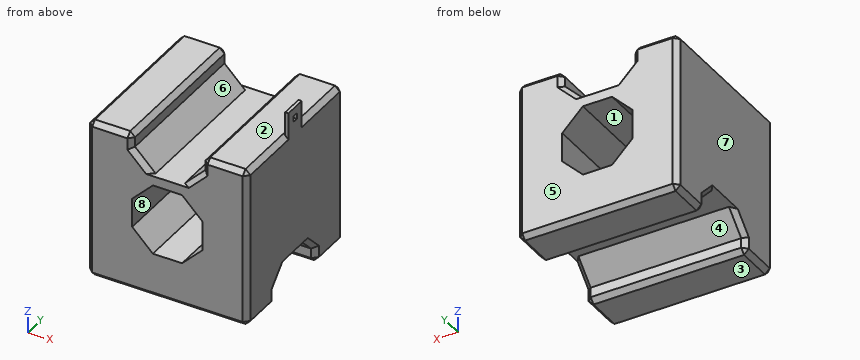
```python
from build123d import *

# Parameters (mm, degrees)
SKETCH1_W                = 50
SKETCH1_H                = 50
BOSS_EXTRUDE1_DEPTH      = 50
CUT_EXTRUDE2_DEPTH       = 87.602540378
CUT_EXTRUDE3_DEPTH       = 87.602540378
CHAMFER1_SIZE            = 1.5
BOSS_EXTRUDE2_DEPTH      = 7
BOSS_EXTRUDE2_DEPTH_BACK = 10
SKETCH5_W                = 1
SKETCH5_H                = 7
SKETCH6_W                = 1.8
SKETCH6_H                = 1.8
CUT_EXTRUDE4_DEPTH       = 7


with BuildPart() as part:
    # Sketch1 → Boss-Extrude1 (new body)
    with BuildSketch(Plane.XY):
        with Locations((25, 25)):
            Rectangle(SKETCH1_W, SKETCH1_H)
    extrude(amount=BOSS_EXTRUDE1_DEPTH)

    # Sketch3 → Cut-Extrude2 (cut, through all)
    with BuildSketch(Plane.XZ):
        Polygon((29.556349186, 36), (20.443650814, 36), (14, 29.556349186), (14, 20.443650814), (20.443650814, 14), (29.556349186, 14), (36, 20.443650814), (36, 29.556349186), align=None)
        Polygon((29.556349186, 39), (36, 45.443650814), (36, 54.556349186), (29.556349186, 61), (20.443650814, 61), (14, 54.556349186), (14, 45.443650814), (20.443650814, 39), align=None)
    extrude(amount=-CUT_EXTRUDE2_DEPTH, mode=Mode.SUBTRACT)

    # Sketch4 → Cut-Extrude3 (cut, through all)
    with BuildSketch(Plane.ZY):
        Polygon((4.556349186, 14), (11, 20.443650814), (11, 29.556349186), (4.556349186, 36), (-4.556349186, 36), (-11, 29.556349186), (-11, 20.443650814), (-4.556349186, 14), align=None)
    extrude(amount=-CUT_EXTRUDE3_DEPTH, mode=Mode.SUBTRACT)

    # Chamfer1
    chamfer1_edges = [part.edges().sort_by_distance(p)[0] for p in [
        (50, 25, 50),
        (43, 50, 50),
        (43, 0, 50),
        (7, 50, 50),
        (36, 25, 50),
        (14, 25, 50),
        (0, 25, 50),
        (14, 50, 47.721825407),
        (36, 50, 47.721825407),
        (25, 50, 0),
        (36, 0, 47.721825407),
        (14, 0, 47.721825407),
        (17.221825407, 0, 42.221825407),
        (32.778174593, 0, 42.221825407),
        (17.221825407, 50, 42.221825407),
        (50, 7, 0),
        (32.778174593, 50, 42.221825407),
        (25, 0, 0),
        (0, 43, 0),
        (7, 0, 50),
        (0, 50, 25),
        (50, 50, 25),
        (50, 0, 25),
        (0, 0, 25),
        (0, 7, 0),
        (50, 43, 0),
        (25, 36, 0),
        (25, 14, 0),
        (50, 14, 2.278174593),
        (50, 36, 2.278174593),
        (50, 32.778174593, 7.778174593),
        (50, 17.221825407, 7.778174593),
        (0, 14, 2.278174593),
        (0, 17.221825407, 7.778174593),
        (0, 32.778174593, 7.778174593),
        (0, 36, 2.278174593),
    ]]
    chamfer(chamfer1_edges, length=CHAMFER1_SIZE)

    # Sketch5 → Boss-Extrude2 (add, two sides: drawn at the far end of the back side and taken through both)
    with BuildSketch(Plane.XY.offset(50).offset(-BOSS_EXTRUDE2_DEPTH_BACK)):
        with Locations((49.5, 25)):
            Rectangle(SKETCH5_W, SKETCH5_H)
    extrude(amount=BOSS_EXTRUDE2_DEPTH + BOSS_EXTRUDE2_DEPTH_BACK)

    # Sketch6 → Cut-Extrude4 (cut)
    with BuildSketch(Plane(origin=(50, 0, 0), x_dir=(0, 0, -1), z_dir=(1, 0, 0))):
        with Locations((-53.6, 25)):
            Rectangle(SKETCH6_W, SKETCH6_H)
    extrude(amount=-CUT_EXTRUDE4_DEPTH, mode=Mode.SUBTRACT)


solid = part.part
```
Work out the finished part from the listing and answer in its coordinate system (mm). Face numbers are marked on the shaded views. A direction names the side the tool comes from. Give positions to 0.01 mm unless a question says otherwise; leave off trailing zeros. Write each loop counter-clockwise with the first axis right and the second up, starting at its lowest first coordinate (ties: lowest second). Pieces come first, ordered by that corner, then holes.
(1) The part is cut by section C-C on z = 27. Write down the section's boundary in (x, y).
Final values:
outline: (0, 1.5) - (1.5, 0) - (14, 0) - (14, 50) - (1.5, 50) - (0, 48.5) - close; (36, 0) - (48.5, 0) - (50, 1.5) - (50, 48.5) - (48.5, 50) - (36, 50) - close
(2) Straight lines are drawn through the part: line 1 (Y direction, x = 12.5, z = 2.5); line 2 (Z direction, x = 11.5, y = 41). For each, find the intervals that lie inside material, in ascending order.
Final values:
line 1: y = 0 to 14, 36 to 50
line 2: z = 0 to 50
(3) Flat-ended cylindrical pins translate along their axes: pin 1 Ø2.5 at (x, y) = (27.5, 27) entering from +Z; pin 2 Ø2 at (y, z) = (26, 53.5) entering from -X; pin 3 Ø10.5 at (x, y) = (27, 22) entering from +Z. Find the tip coordinate at first contact, or state that the pin passes through.
Final values:
pin 1: stops at z = 39
pin 2: stops at x = 49
pin 3: stops at z = 41.69
(4) The part is cut by section D-D on y = 4. Write down the section's boundary in (x, z).
Final values:
outline: (0, 1.5) - (1.5, 0) - (48.5, 0) - (50, 1.5) - (50, 48.5) - (48.5, 50) - (37.5, 50) - (36, 48.5) - (36, 45.44) - (29.56, 39) - (20.44, 39) - (14, 45.44) - (14, 48.5) - (12.5, 50) - (1.5, 50) - (0, 48.5) - close; hole (14, 20.44) - (20.44, 14) - (29.56, 14) - (36, 20.44) - (36, 29.56) - (29.56, 36) - (20.44, 36) - (14, 29.56) - close
(5) Which of the six approach directions +Z, -Z, +X, -X, +Y, -Y give full straight-line access (tool end or side, diameter ignored) to the marked faces 4, 5, 6, 7 and 8?
Final values:
face 4: -Z, +X, -X
face 5: +Z, -Z, +X, -X, +Y
face 6: +Z, +Y, -Y
face 7: +Z, -Z, -X, +Y, -Y
face 8: +Y, -Y
(6) The part is cut by section A-A on y = 25. Write down the section's boundary in (x, z), plus the area to 3 significant figures.
Final values:
outline: (0, 11) - (50, 11) - (50, 52.7) - (49, 52.7) - (49, 49.5) - (48.5, 50) - (37.5, 50) - (36, 48.5) - (36, 45.44) - (29.56, 39) - (20.44, 39) - (14, 45.44) - (14, 48.5) - (12.5, 50) - (1.5, 50) - (0, 48.5) - close; (49, 54.5) - (50, 54.5) - (50, 57) - (49, 57) - close; hole (14, 20.44) - (20.44, 14) - (29.56, 14) - (36, 20.44) - (36, 29.56) - (29.56, 36) - (20.44, 36) - (14, 29.56) - close
area: 1,350 mm2
(7) The part is cut by section B-B on x = 28.5. Write down the section's boundary in (y, z), plus the area to 3 significant figures.
Final values:
outline: (0, 1.5) - (1.5, 0) - (12.5, 0) - (14, 1.5) - (14, 4.56) - (20.44, 11) - (29.56, 11) - (36, 4.56) - (36, 1.5) - (37.5, 0) - (48.5, 0) - (50, 1.5) - (50, 14) - (0, 14) - close; (0, 36) - (50, 36) - (50, 39) - (0, 39) - close
area: 645 mm2
(8) The mould has two halves that part along Z. Classify the marked faces 1, 2 and 3: pulls with the +Z half, pulls with the -Z half, needs draft (parallel to the pull), parting line crosses it, or undercut.
Final values:
face 1: undercut
face 2: pulls with the +Z half
face 3: pulls with the -Z half
